Part model, mm, in its own coordinate system. Face numbers are marked on the shaded views. Give positions to 0.01 mm unless a question says otherwise; leave off trailing zeros. Loops run counter-clockwise (first coordinate to the right, second up) from the corner with the lowest first, then second, coordinate; pieces in that order, holes last. Notation, with made-up numbers: M 29,-36.75 L 63,-36.75 A26 cw 63,-20.75 Z; hole C 26,11.5 d5. An arc over 180 degrees is marked long. Answer in a Markdown table with one row per item.
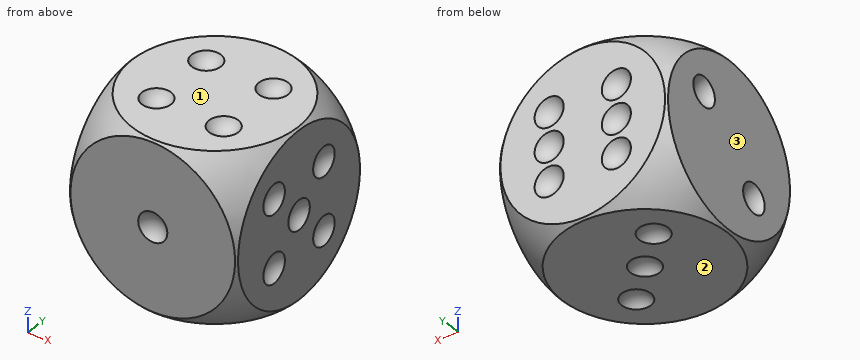
from build123d import *

# Parameters (mm, degrees)
FUSION003_PLACEMENT_ANGLE = 90
FUSION001_PLACEMENT_ANGLE = 270
FUSION002_PLACEMENT_ANGLE = 270
FUSION_PLACEMENT_ANGLE    = 90
BOX_W                     = 10
BOX_H                     = 10
BOX_DEPTH                 = 10


with BuildPart() as sphere013:
    # Sphere014 → Sphere014 (revolve)
    with BuildSketch(Plane(origin=(3, 0, 3), x_dir=(1, 0, 0), z_dir=(0, -1, 0))):
        with BuildLine():
            ThreePointArc((0, -1), (1, 0), (0, 1))
            Line((0, 1), (0, -1))
        make_face()
    revolve(axis=Axis((3, 0, 3), (0, 0, 1)))


with BuildPart() as sphere012:
    # Sphere013 → Sphere013 (revolve)
    with BuildSketch(Plane(origin=(3, 0, 7), x_dir=(1, 0, 0), z_dir=(0, -1, 0))):
        with BuildLine():
            ThreePointArc((0, -1), (1, 0), (0, 1))
            Line((0, 1), (0, -1))
        make_face()
    revolve(axis=Axis((3, 0, 7), (0, 0, 1)))


with BuildPart() as sphere011:
    # Sphere012 → Sphere012 (revolve)
    with BuildSketch(Plane(origin=(7, 0, 3), x_dir=(1, 0, 0), z_dir=(0, -1, 0))):
        with BuildLine():
            ThreePointArc((0, -1), (1, 0), (0, 1))
            Line((0, 1), (0, -1))
        make_face()
    revolve(axis=Axis((7, 0, 3), (0, 0, 1)))


with BuildPart() as sphere010:
    # Sphere011 → Sphere011 (revolve)
    with BuildSketch(Plane(origin=(7, 0, 7), x_dir=(1, 0, 0), z_dir=(0, -1, 0))):
        with BuildLine():
            ThreePointArc((0, -1), (1, 0), (0, 1))
            Line((0, 1), (0, -1))
        make_face()
    revolve(axis=Axis((7, 0, 7), (0, 0, 1)))


with BuildPart() as side5:
    # Sphere015 → Sphere015 (revolve)
    with BuildSketch(Plane(origin=(5, 0, 5), x_dir=(1, 0, 0), z_dir=(0, -1, 0))):
        with BuildLine():
            ThreePointArc((0, -1), (1, 0), (0, 1))
            Line((0, 1), (0, -1))
        make_face()
    revolve(axis=Axis((5, 0, 5), (0, 0, 1)))

    # Fusion003: union Sphere013, Sphere012, Sphere011, Sphere010
    add(sphere013.part)
    add(sphere012.part)
    add(sphere011.part)
    add(sphere010.part)


with BuildPart() as side5_1:
    # Fusion003 placement: moved
    add(side5.part.moved(Location((10.5, 0, 0))).rotate(Axis((10.5, 0, 0), (0, 0, 1)), FUSION003_PLACEMENT_ANGLE))


with BuildPart() as side1:
    # Sphere001 → Sphere001 (revolve)
    with BuildSketch(Plane(origin=(5, -0.5, 5), x_dir=(1, 0, 0), z_dir=(0, -1, 0))):
        with BuildLine():
            ThreePointArc((0, -1), (1, 0), (0, 1))
            Line((0, 1), (0, -1))
        make_face()
    revolve(axis=Axis((5, -0.5, 5), (0, 0, 1)))


with BuildPart() as sphere004:
    # Sphere005 → Sphere005 (revolve)
    with BuildSketch(Plane(origin=(3, 0, 7), x_dir=(1, 0, 0), z_dir=(0, -1, 0))):
        with BuildLine():
            ThreePointArc((0, -1), (1, 0), (0, 1))
            Line((0, 1), (0, -1))
        make_face()
    revolve(axis=Axis((3, 0, 7), (0, 0, 1)))


with BuildPart() as sphere003:
    # Sphere004 → Sphere004 (revolve)
    with BuildSketch(Plane(origin=(5, 0, 5), x_dir=(1, 0, 0), z_dir=(0, -1, 0))):
        with BuildLine():
            ThreePointArc((0, -1), (1, 0), (0, 1))
            Line((0, 1), (0, -1))
        make_face()
    revolve(axis=Axis((5, 0, 5), (0, 0, 1)))


with BuildPart() as side3:
    # Sphere006 → Sphere006 (revolve)
    with BuildSketch(Plane(origin=(7, 0, 3), x_dir=(1, 0, 0), z_dir=(0, -1, 0))):
        with BuildLine():
            ThreePointArc((0, -1), (1, 0), (0, 1))
            Line((0, 1), (0, -1))
        make_face()
    revolve(axis=Axis((7, 0, 3), (0, 0, 1)))

    # Fusion001: union Sphere004, Sphere003
    add(sphere004.part)
    add(sphere003.part)


with BuildPart() as side3_1:
    # Fusion001 placement: moved
    add(side3.part.moved(Location((0, 0, -0.5))).rotate(Axis((0, 0, -0.5), (1, 0, 0)), FUSION001_PLACEMENT_ANGLE))


with BuildPart() as sphere008:
    # Sphere009 → Sphere009 (revolve)
    with BuildSketch(Plane(origin=(3, 0, 7), x_dir=(1, 0, 0), z_dir=(0, -1, 0))):
        with BuildLine():
            ThreePointArc((0, -1), (1, 0), (0, 1))
            Line((0, 1), (0, -1))
        make_face()
    revolve(axis=Axis((3, 0, 7), (0, 0, 1)))


with BuildPart() as sphere007:
    # Sphere008 → Sphere008 (revolve)
    with BuildSketch(Plane(origin=(7, 0, 3), x_dir=(1, 0, 0), z_dir=(0, -1, 0))):
        with BuildLine():
            ThreePointArc((0, -1), (1, 0), (0, 1))
            Line((0, 1), (0, -1))
        make_face()
    revolve(axis=Axis((7, 0, 3), (0, 0, 1)))


with BuildPart() as sphere006:
    # Sphere007 → Sphere007 (revolve)
    with BuildSketch(Plane(origin=(7, 0, 7), x_dir=(1, 0, 0), z_dir=(0, -1, 0))):
        with BuildLine():
            ThreePointArc((0, -1), (1, 0), (0, 1))
            Line((0, 1), (0, -1))
        make_face()
    revolve(axis=Axis((7, 0, 7), (0, 0, 1)))


with BuildPart() as side4:
    # Sphere010 → Sphere010 (revolve)
    with BuildSketch(Plane(origin=(3, 0, 3), x_dir=(1, 0, 0), z_dir=(0, -1, 0))):
        with BuildLine():
            ThreePointArc((0, -1), (1, 0), (0, 1))
            Line((0, 1), (0, -1))
        make_face()
    revolve(axis=Axis((3, 0, 3), (0, 0, 1)))

    # Fusion002: union Sphere008, Sphere007, Sphere006
    add(sphere008.part)
    add(sphere007.part)
    add(sphere006.part)


with BuildPart() as side4_1:
    # Fusion002 placement: moved
    add(side4.part.moved(Location((0, 0, 10.5))).rotate(Axis((0, 0, 10.5), (1, 0, 0)), FUSION002_PLACEMENT_ANGLE))


with BuildPart() as sphere001:
    # Sphere002 → Sphere002 (revolve)
    with BuildSketch(Plane(origin=(7, 0, 7), x_dir=(1, 0, 0), z_dir=(0, -1, 0))):
        with BuildLine():
            ThreePointArc((0, -1), (1, 0), (0, 1))
            Line((0, 1), (0, -1))
        make_face()
    revolve(axis=Axis((7, 0, 7), (0, 0, 1)))


with BuildPart() as side2:
    # Sphere003 → Sphere003 (revolve)
    with BuildSketch(Plane(origin=(3, 0, 3), x_dir=(1, 0, 0), z_dir=(0, -1, 0))):
        with BuildLine():
            ThreePointArc((0, -1), (1, 0), (0, 1))
            Line((0, 1), (0, -1))
        make_face()
    revolve(axis=Axis((3, 0, 3), (0, 0, 1)))

    # Fusion: union Sphere001
    add(sphere001.part)


with BuildPart() as side2_1:
    # Fusion placement: moved
    add(side2.part.moved(Location((-0.5, 0, 0))).rotate(Axis((-0.5, 0, 0), (0, 0, 1)), FUSION_PLACEMENT_ANGLE))


with BuildPart() as sphere019:
    # Sphere020 → Sphere020 (revolve)
    with BuildSketch(Plane(origin=(3, 0, 5), x_dir=(1, 0, 0), z_dir=(0, -1, 0))):
        with BuildLine():
            ThreePointArc((0, -1), (1, 0), (0, 1))
            Line((0, 1), (0, -1))
        make_face()
    revolve(axis=Axis((3, 0, 5), (0, 0, 1)))


with BuildPart() as sphere018:
    # Sphere019 → Sphere019 (revolve)
    with BuildSketch(Plane(origin=(3, 0, 3), x_dir=(1, 0, 0), z_dir=(0, -1, 0))):
        with BuildLine():
            ThreePointArc((0, -1), (1, 0), (0, 1))
            Line((0, 1), (0, -1))
        make_face()
    revolve(axis=Axis((3, 0, 3), (0, 0, 1)))


with BuildPart() as sphere017:
    # Sphere018 → Sphere018 (revolve)
    with BuildSketch(Plane(origin=(3, 0, 7), x_dir=(1, 0, 0), z_dir=(0, -1, 0))):
        with BuildLine():
            ThreePointArc((0, -1), (1, 0), (0, 1))
            Line((0, 1), (0, -1))
        make_face()
    revolve(axis=Axis((3, 0, 7), (0, 0, 1)))


with BuildPart() as sphere016:
    # Sphere017 → Sphere017 (revolve)
    with BuildSketch(Plane(origin=(7, 0, 3), x_dir=(1, 0, 0), z_dir=(0, -1, 0))):
        with BuildLine():
            ThreePointArc((0, -1), (1, 0), (0, 1))
            Line((0, 1), (0, -1))
        make_face()
    revolve(axis=Axis((7, 0, 3), (0, 0, 1)))


with BuildPart() as sphere015:
    # Sphere016 → Sphere016 (revolve)
    with BuildSketch(Plane(origin=(7, 0, 7), x_dir=(1, 0, 0), z_dir=(0, -1, 0))):
        with BuildLine():
            ThreePointArc((0, -1), (1, 0), (0, 1))
            Line((0, 1), (0, -1))
        make_face()
    revolve(axis=Axis((7, 0, 7), (0, 0, 1)))


with BuildPart() as sides:
    # Sphere021 → Sphere021 (revolve)
    with BuildSketch(Plane(origin=(7, 0, 5), x_dir=(1, 0, 0), z_dir=(0, -1, 0))):
        with BuildLine():
            ThreePointArc((0, -1), (1, 0), (0, 1))
            Line((0, 1), (0, -1))
        make_face()
    revolve(axis=Axis((7, 0, 5), (0, 0, 1)))

    # Fusion004: union Sphere019, Sphere018, Sphere017, Sphere016, Sphere015
    add(sphere019.part)
    add(sphere018.part)
    add(sphere017.part)
    add(sphere016.part)
    add(sphere015.part)


with BuildPart() as sides_1:
    # Fusion004 placement: moved
    add(sides.part.moved(Location((0, 10.5, 0))))

    # Fusion005: union Side5, Side1, Side3, Side4, Side2
    add(side5_1.part)
    add(side1.part)
    add(side3_1.part)
    add(side4_1.part)
    add(side2_1.part)


with BuildPart() as sphere:
    # Sphere → Sphere (revolve)
    with BuildSketch(Plane(origin=(5, 5, 5), x_dir=(1, 0, 0), z_dir=(0, -1, 0))):
        with BuildLine():
            ThreePointArc((0, -7), (7, 0), (0, 7))
            Line((0, 7), (0, -7))
        make_face()
    revolve(axis=Axis((5, 5, 5), (0, 0, 1)))


with BuildPart() as dice:
    # Box → Box (new body)
    with BuildSketch(Plane.XY):
        with Locations((5, 5)):
            Rectangle(BOX_W, BOX_H)
    extrude(amount=BOX_DEPTH)

    # Common: intersect Sphere
    add(sphere.part, mode=Mode.INTERSECT)

    # Cut: cut Sides
    add(sides_1.part, mode=Mode.SUBTRACT)


solid = dice.part
(1) Saw through at C-C (y = 2.5). Write the cut outline in (x, z).
Recorded:
| item | result |
|---|---|
| outline | M 0,0.79 A6.54 ccw 0.79,0 L 6.29,0 A0.87 cw 7.71,0 L 9.21,0 A6.54 ccw 10,0.79 L 10,2.29 A0.87 cw 10,3.71 L 10,6.29 A0.87 cw 10,7.71 L 10,9.21 A6.54 ccw 9.21,10 L 7.71,10 A0.87 cw 6.29,10 L 3.71,10 A0.87 cw 2.29,10 L 0.79,10 A6.54 ccw 0,9.21 L 0,3.71 A0.87 cw 0,2.29 Z |
(2) Saw through at B-B (x = 1). Write the cut outline in (y, z).
Recorded:
| item | result |
|---|---|
| outline | M 0,2.17 A5.74 ccw 2.17,0 L 7.83,0 A5.74 ccw 10,2.17 L 10,7.83 A5.74 ccw 7.83,10 L 2.17,10 A5.74 ccw 0,7.83 Z |
(3) Saw through at A-A (z = 9.75). Write the cut outline in (x, y).
Recorded:
| item | result |
|---|---|
| outline | M 0,3.8 A5.14 ccw 3.8,0 L 6.2,0 A5.14 ccw 10,3.8 L 10,6.2 A5.14 ccw 6.2,10 L 3.8,10 A5.14 ccw 0,6.2 Z; hole C 3,3 d1.32; hole C 3,7 d1.32; hole C 7,3 d1.32; hole C 7,7 d1.32 |
(4) Pull direction Z, two halves, no side cores. Call the marked faces 1, 2 and 3: +Z half, -Z half, draft (parallel to the pull), parting line (faces both ways), or undercut.
Recorded:
| item | result |
|---|---|
| face 1 | +Z half |
| face 2 | -Z half |
| face 3 | draft |
(5) Drill centre lines: line 1 along Z through (x, y) = (9.75, 7.25); line 2 along Y through (x, z) = (1, 8); line 3 along X through (y, z) = (6.25, 3.25). Where is each one in solid material? Low to high.
Recorded:
| item | result |
|---|---|
| line 1 | z = 0.38 to 2.39, 3.61 to 6.39, 7.61 to 9.62 |
| line 2 | y = 0.1 to 9.9 |
| line 3 | x = 0 to 9.89 |
